```python
from build123d import *

# Parameters (mm, degrees)
BOSS_EXTRUDE1_DEPTH = 7
SKETCH3_R           = 2.5
CUT_EXTRUDE1_DEPTH  = 6
FILLET2_R           = 0.5
CHAMFER1_SIZE       = 1


with BuildPart() as part:
    # Sketch1 → Boss-Extrude1 (new, symmetric)
    with BuildSketch(Plane(origin=(0, 0, 0), x_dir=(0, 0, -1), z_dir=(1, 0, 0))):
        with BuildLine():
            Line((-21, 0), (21, 0))
            Line((21, 0), (21, 6))
            Line((21, 6), (9, 6))
            Line((9, 6), (9, 32.8))
            Line((9, 32.8), (0.5, 32.8))
            Line((0.5, 32.8), (0.5, 23.968626967))
            ThreePointArc((0.5, 23.968626967), (0, 16), (-0.5, 23.968626967))
            Line((-0.5, 23.968626967), (-0.5, 32.8))
            Line((-0.5, 32.8), (-9, 32.8))
            Line((-9, 32.8), (-9, 6))
            Line((-9, 6), (-21, 6))
            Line((-21, 6), (-21, 0))
        make_face()
    extrude(amount=BOSS_EXTRUDE1_DEPTH, both=True)

    # Sketch3 → Cut-Extrude1 (cut)
    with BuildSketch(Plane(origin=(0, 6, 0), x_dir=(1, 0, 0), z_dir=(0, 1, 0))):
        with Locations(Location((0, 16, 0), (0, 0, 270))):
            Circle(SKETCH3_R)
        with Locations(Location((0, -16, 0), (0, 0, 270))):
            Circle(SKETCH3_R)
    extrude(amount=-CUT_EXTRUDE1_DEPTH, mode=Mode.SUBTRACT)

    # Fillet2
    fillet2_edges = [part.edges().sort_by_distance(p)[0] for p in [
        (-7, 6, 15),
        (-7, 19.4, 9),
        (7, 3, -21),
        (-7, 32.8, 4.75),
        (-7, 28.384313483, 0.5),
        (-7, 16, 0),
        (-7, 28.384313483, -0.5),
        (-7, 32.8, -4.75),
        (-7, 19.4, -9),
        (-7, 6, -15),
        (-7, 3, -21),
        (-7, 3, 21),
        (7, 6, -15),
        (0, 6, 21),
        (0, 6, 9),
        (0, 32.8, 9),
        (7, 19.4, -9),
        (0, 32.8, 0.5),
        (0, 23.968626967, 0.5),
        (0, 23.968626967, -0.5),
        (0, 32.8, -0.5),
        (0, 32.8, -9),
        (0, 6, -9),
        (0, 6, -21),
        (7, 32.8, -4.75),
        (7, 28.384313483, -0.5),
        (7, 16, 0),
        (7, 28.384313483, 0.5),
        (7, 32.8, 4.75),
        (7, 19.4, 9),
        (7, 6, 15),
        (7, 3, 21),
    ]]
    fillet(fillet2_edges, radius=FILLET2_R)

    # Chamfer1
    chamfer1_edges = [part.edges().sort_by_distance(p)[0] for p in [
        (0, 6, -18.5),
        (0, 6, 13.5),
    ]]
    chamfer(chamfer1_edges, length=CHAMFER1_SIZE)


solid = part.part
```
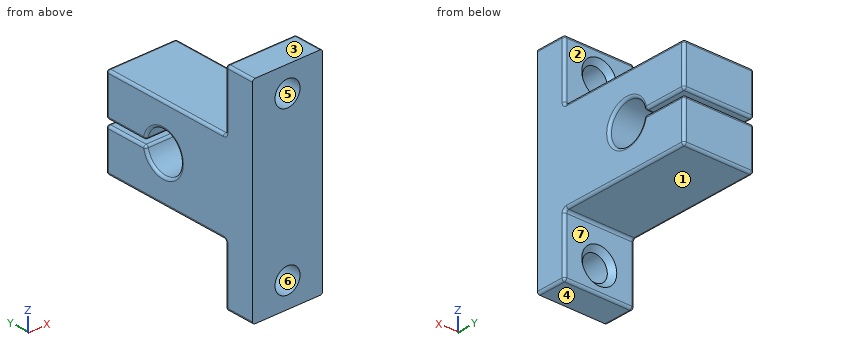
Could you check a few things on this model? Use its own coordinates, in mm. Face numbers are marked on the shaded views. A direction names the side the tool comes from. Coordinates: 2 decimals unless noted, no trailing zeros. Write each loop counter-clockwise with the first axis right and the second up, starting at its lowest first coordinate (ties: lowest second). Pieces come first, ordered by that corner, then holes. Notation, with made-up numbers: M -9,7 L 4,7 A13 ccw 4,20 Z; hole C -31,62.5 d6. An arc over 180 degrees is marked long. Answer as CSV lines item,"result". Start each with the question number.
1) Please list where these lines run through material, in increasing order: line 1 (Z direction, x = 0, y = 26.5); line 2 (X direction, y = 3.5, z = 16); line 3 (Z direction, x = 3.75, y = 20). Write a range as from..to.
2) For the marked faces 1, 2 and 3, which set-ups out of +Z, -Z, +X, -X, +Y, -Y let a thin tool reach every point of the face, with its end or its side?
3) We'd pull the mould along Z, two halves only. Please class the marked faces 4, 5, 6 and 7: +Z half, -Z half, draft (parallel to the pull), parting line (faces both ways), or undercut.
4) I want a section at C-C, the plane z = 0. Please give me the cut outline in (x, y), and give its area (3 significant figures).
5) I want a section at B-B, the plane x = 0. Give the number of separate pieces and of enclosed holes in the cut face, and give its area (3 significant figures).
6) I want a section at D-D, the plane x = -4. Please give me the cut outline in (y, z), and give its area (3 significant figures).
7) I want a section at A-A, the plane z = 16. Please give me the cut outline in (x, y), and give its area (3 significant figures).
8) For P1, Ø1.5, axis at x = -5, y = 24, coming from the +Z side; P2, Ø4, axis at x = 0, z = -16, coming from the -Y side; P3, Ø8, axis at x = 0, z = 16, coming from the +Y side, each with a flat end and sliding along its axis, tell me the tip position at first contact or that it passes through.
Data:
1,line 1,"z = -9..-0.5, 0.5..9"
1,line 2,"x = -7..-2.5, 2.5..7"
1,line 3,"z = -9..-4, 4..9"
2,face 1,"-Z, +X, -X, +Y"
2,face 2,"+Z, +X, -X, +Y"
2,face 3,"+Z, +X, -X, +Y, -Y"
3,face 4,"-Z half"
3,face 5,"undercut"
3,face 6,"undercut"
3,face 7,"draft"
4,outline,"M -7,0 L 7,0 L 7,15.5 A0.5 ccw 6.5,16 L -6.5,16 A0.5 ccw -7,15.5 Z"
4,area,"224 mm^2"
5,separate pieces,"3"
5,enclosed holes,"0"
5,area,"613 mm^2"
6,outline,"M 0,-21 L 5.5,-21 A0.5 ccw 6,-20.5 L 6,-9.5 A0.5 cw 6.5,-9 L 32.3,-9 A0.5 ccw 32.8,-8.5 L 32.8,-1 A0.5 ccw 32.3,-0.5 L 24.39,-0.5 A0.5 ccw 23.9,-0.89 A4 cw long 23.9,0.89 A0.5 ccw 24.39,0.5 L 32.3,0.5 A0.5 ccw 32.8,1 L 32.8,8.5 A0.5 ccw 32.3,9 L 6.5,9 A0.5 cw 6,9.5 L 6,20.5 A0.5 ccw 5.5,21 L 0,21 Z"
6,area,"675 mm^2"
7,outline,"M -7,0 L -2.5,0 L -2.5,5 L -3.5,6 L -6.5,6 A0.5 ccw -7,5.5 Z; M 2.5,0 L 7,0 L 7,5.5 A0.5 ccw 6.5,6 L 3.5,6 L 2.5,5 Z"
7,area,"52.9 mm^2"
8,P1,"stops at z = 9"
8,P2,"passes through"
8,P3,"stops at y = 6"
